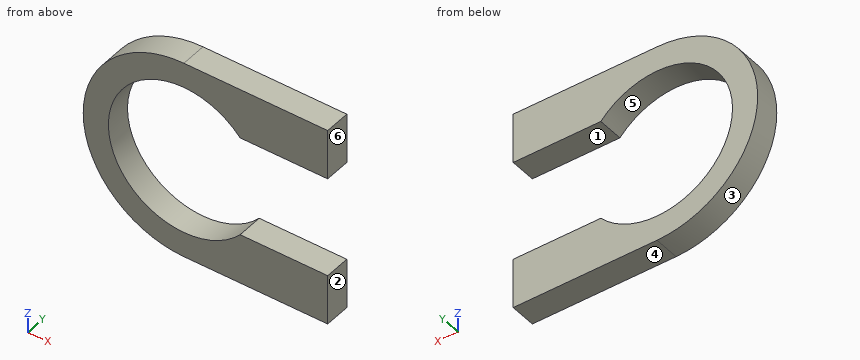
```python
from build123d import *

# Parameters (mm, degrees)
PAD_DEPTH = 1.8


with BuildPart() as part:
    # Sketch → Pad (new body)
    with BuildSketch(Plane.XZ):
        with BuildLine():
            ThreePointArc((3.91, 3.503484), (-5.25, 0), (3.91, -3.503484))
            Line((10, -3.503484), (3.91, -3.503484))
            Line((10, -3.503484), (10, -7))
            Line((10, -7), (0, -7))
            ThreePointArc((0, 7), (-7, 0), (0, -7))
            Line((0, 7), (10, 7))
            Line((10, 7), (10, 3.503484))
            Line((3.91, 3.503484), (10, 3.503484))
        make_face()
    extrude(amount=PAD_DEPTH)


solid = part.part
```
Input: part model. Units: mm. Frame: model coordinates. Face numbers are marked on the shaded views. A direction names the side the tool comes from. Coordinates: 2 decimals unless noted, no trailing zeros. Write each loop counter-clockwise with the first axis right and the second up, starting at its lowest first coordinate (ties: lowest second). Pieces come first, ordered by that corner, then holes.
1) Section D-D on z = 0. Output: boundary loops of the cut face in (x, y).
2) Mould query, pull axis X, two halves, no side actions, for the marked faces 3, 4, 5 and 6. Classes: pulls with the +X half, pulls with the -X half, needs draft (parallel to the pull), parting line crosses it, or undercut.
3) Material intervals for line 1 along Z through (x, y) = (8, -0.55); line 2 along Z through (x, y) = (0, -1.4); line 3 along X through (y, z) = (-1.35, 0), sorted ascending.
4) Pin query (flat end, axial travel): pin 1 Ø6.5 at (x, z) = (0, 0) entering from -Y. Return the tip coordinate at first contact, or that it passes through.
5) Section A-A on x = 1. Output: boundary loops of the cut face in (y, z).
6) Section C-C on x = 6.75. Output: boundary loops of the cut face in (y, z), and give its area (3 significant figures).
7) Section B-B on y = -1. Output: boundary loops of the cut face in (x, z), and give its area (3 significant figures).
8) Set-up query: the marked faces 1 and 2. Return all of +Z, -Z, +X, -X, +Y, -Y with unobstructed straight access to the full face (end or side cutting, diameter ignored); none if empty.
Check result:
1. outline: (-7, -1.8) - (-5.25, -1.8) - (-5.25, 0) - (-7, 0) - close
2. face 3: pulls with the -X half
2. face 4: needs draft
2. face 5: undercut
2. face 6: pulls with the +X half
3. line 1: z = -7 to -3.5, 3.5 to 7
3. line 2: z = -7 to -5.25, 5.25 to 7
3. line 3: x = -7 to -5.25
4. pin 1: passes through
5. outline: (-1.8, -7) - (0, -7) - (0, -5.15) - (-1.8, -5.15) - close; (-1.8, 5.15) - (0, 5.15) - (0, 7) - (-1.8, 7) - close
6. outline: (-1.8, -7) - (0, -7) - (0, -3.5) - (-1.8, -3.5) - close; (-1.8, 3.5) - (0, 3.5) - (0, 7) - (-1.8, 7) - close
6. area: 12.6 mm2
7. outline: (0, -7) - (10, -7) - (10, -3.5) - (3.91, -3.5) arc R5.25 cw (long way) to (3.91, 3.5) - (10, 3.5) - (10, 7) - (0, 7) arc R7 ccw to start
7. area: 94.1 mm2
8. face 1: +X, +Y, -Y
8. face 2: +Z, -Z, +X, +Y, -Y
